Autodesk Inventor part; units mm, degrees
ref_plane "bracket_to_bolt_XY" through (1, 10, 0) normal (0, 0, 1) x (1, 0, 0)
ref_plane "bracket_to_bolt_YZ" through (1, 10, 0) normal (1, 0, 0) x (0, 1, 0)
ref_plane "bracket_to_bolt_ZX" through (1, 10, 0) normal (0, 1, 0) x (0, 0, 1)
sketch "Sketch_15" plane through (0, 0, 0) normal (1, 0, 0) x (0, 1, 0)
  line L0 (4.0858, 30) -> (0, 30)
  line L1 (0, 30) -> (0, 0)
  line L2 (0, 0) -> (30, 0)
  line L3 (30, 0) -> (30, 4.0858)
  arc A0 (30, 4.0858) -> (29.7071, 4.7929) centre (29, 4.0858) ccw
  line L4 (29.7071, 4.7929) -> (4.7929, 29.7071)
  arc A1 (4.7929, 29.7071) -> (4.0858, 30) centre (4.0858, 29) ccw
extrude "Extrusion1" add sketch "Sketch_15" along normal mid plane 20
sketch "Sketch_16" plane through (0, 0, 0) normal (1, 0, 0) x (0, 1, 0)
  line L0 (34.5, 34.5) -> (2.9278, 34.5)
  line L1 (2.9278, 34.5) -> (4.5, 4.5)
  line L2 (4.5, 4.5) -> (34.5, 4.5)
  line L3 (34.5, 4.5) -> (34.5, 34.5)
extrude "Extrusion2" cut sketch "Sketch_16" along normal mid plane 15
sketch "Sketch_17" plane through (0, 4.5, 0) normal (0, 1, 0) x (1, 0, 0)
  line L0 (-5.4209, -10.5) -> (-4.4687, -18.5299)
  arc A0 (-4.4687, -18.5299) -> (4.4687, -18.5299) centre (0, -18) ccw
  line L1 (4.4687, -18.5299) -> (5.4209, -10.5)
  line L2 (5.4209, -10.5) -> (-5.4209, -10.5)
extrude "Extrusion3" add sketch "Sketch_17" against normal blind 2.25
sketch "Sketch_18" plane through (0, 12, 0) normal (0, 1, 0) x (1, 0, 0)
  line L0 (7.5, -12) -> (10, -12)
  line L1 (10, -12) -> (10, -14.5)
  line L2 (10, -14.5) -> (9.567, -14.067)
  line L3 (9.567, -14.067) -> (7.933, -14.067)
  line L4 (7.933, -14.067) -> (7.5, -14.5)
  line L5 (7.5, -14.5) -> (7.5, -12)
  line L6 (7.5, -12) -> (10, -12)
revolve "Revolution1" cut sketch "Sketch_18" angle 360 about axis through (7.5, 12, 12) along (-1, 0, 0)
thread "Thread1"
sketch "Sketch_19" plane through (0, 12, 0) normal (0, 1, 0) x (1, 0, 0)
  line L0 (-10, -12) -> (-7.5, -12)
  line L1 (-7.5, -12) -> (-7.5, -14.5)
  line L2 (-7.5, -14.5) -> (-7.933, -14.067)
  line L3 (-7.933, -14.067) -> (-9.567, -14.067)
  line L4 (-9.567, -14.067) -> (-10, -14.5)
  line L5 (-10, -14.5) -> (-10, -12)
  line L6 (-10, -12) -> (-7.5, -12)
revolve "Revolution2" cut sketch "Sketch_19" angle 360 about axis through (-10, 12, 12) along (-1, 0, 0)
thread "Thread2"
sketch "Sketch6" plane through (10, 30, 0) normal (0, 0, -1) x (-1, 0, 0)
  point P0 (10, -12)
hole "Hole1" at (0, 18, 0) direction (0, 0, 1) diameter 5.2 depth 4.5
sketch "Sketch7" plane through (10, 30, 0) normal (0, 0, -1) x (-1, 0, 0)
  point P0 (10, -20)
hole "Hole2" at (0, 10, 0) direction (0, 0, 1) diameter 5.2 depth 4.5
sketch "Sketch8" plane through (-10, 0, 0) normal (0, -1, 0) x (1, 0, 0)
  point P0 (10, 18)
hole "Hole3" at (0, 0, 18) direction (0, 1, 0) diameter 5.2 depth 4.5
sketch "Sketch_1" plane through (0, 0, 0) normal (0, 1, 0) x (-1, 0, 0)
  line L0 (10, 30) -> (-10, 30)
  line L1 (-10, 30) -> (-10, 0)
  line L2 (-10, 0) -> (10, 0)
  line L3 (10, 0) -> (10, 30)
extrude "Extrusion4" add sketch "Sketch_1" against normal blind 1
sketch "Sketch_4" plane through (0, 0, 0) normal (0, 1, 0) x (-1, 0, 0)
  line L0 (10, 30) -> (-10, 30)
  line L1 (-10, 30) -> (-10, 0)
  line L2 (-10, 0) -> (10, 0)
  line L3 (10, 0) -> (10, 30)
  line L4 (3, 24.3) -> (3, 26.7)
  arc A0 (3, 26.7) -> (2.7, 27) centre (2.7, 26.7) ccw
  line L5 (2.7, 27) -> (-2.7, 27)
  arc A1 (-2.7, 27) -> (-3, 26.7) centre (-2.7, 26.7) ccw
  line L6 (-3, 26.7) -> (-3, 24.3)
  arc A2 (-3, 24.3) -> (-2.7, 24) centre (-2.7, 24.3) ccw
  line L7 (-2.7, 24) -> (2.7, 24)
  arc A3 (2.7, 24) -> (3, 24.3) centre (2.7, 24.3) ccw
  line L8 (3, 5.3) -> (3, 10.7)
  arc A4 (3, 10.7) -> (2.7, 11) centre (2.7, 10.7) ccw
  line L9 (2.7, 11) -> (-2.7, 11)
  arc A5 (-2.7, 11) -> (-3, 10.7) centre (-2.7, 10.7) ccw
  line L10 (-3, 10.7) -> (-3, 5.3)
  arc A6 (-3, 5.3) -> (-2.7, 5) centre (-2.7, 5.3) ccw
  line L11 (-2.7, 5) -> (2.7, 5)
  arc A7 (2.7, 5) -> (3, 5.3) centre (2.7, 5.3) ccw
extrude "Extrusion5" cut sketch "Sketch_4" against normal blind 1
ref_plane "bracket_to_bolt_XY" through (1, 10, 0) normal (0, 0, 1) x (1, 0, 0)
ref_plane "bracket_to_bolt_YZ" through (1, 10, 0) normal (1, 0, 0) x (0, 1, 0)
ref_plane "bracket_to_bolt_ZX" through (1, 10, 0) normal (0, 1, 0) x (0, 0, 1)
ref_plane "bracket_to_dummy_XY" through (0, 0, 0) normal (0, 1, 0) x (1, 0, 0)
ref_plane "bracket_to_dummy_YZ" through (0, 0, 0) normal (1, 0, 0) x (0, 0, -1)
ref_plane "bracket_to_dummy_ZX" through (0, 0, 0) normal (0, 0, -1) x (0, 1, 0)
ref_plane "to_bolt_4_7_base_XY" through (0, 4.5, 18) normal (0, 1, 0) x (1, 0, 0)
ref_plane "to_bolt_4_7_base_YZ" through (0, 4.5, 18) normal (1, 0, 0) x (0, 0, -1)
ref_plane "to_bolt_4_7_base_ZX" through (0, 4.5, 18) normal (0, 0, -1) x (0, 1, 0)
ref_plane "to_bolt_row_4_to_7_XY" through (0, 18, 4.5) normal (0, 0, 1) x (1, 0, 0)
ref_plane "to_bolt_row_4_to_7_YZ" through (0, 18, 4.5) normal (1, 0, 0) x (0, 1, 0)
ref_plane "to_bolt_row_4_to_7_ZX" through (0, 18, 4.5) normal (0, 1, 0) x (0, 0, 1)
ref_plane "to_nut_base_4_7_XY" through (0, -2, 18) normal (0, 1, 0) x (1, 0, 0)
ref_plane "to_nut_base_4_7_YZ" through (0, -2, 18) normal (1, 0, 0) x (0, 0, -1)
ref_plane "to_nut_base_4_7_ZX" through (0, -2, 18) normal (0, 0, -1) x (0, 1, 0)
ref_plane "to_nut_row_4_to_7_XY" through (0, 18, -2) normal (0, 0, 1) x (1, 0, 0)
ref_plane "to_nut_row_4_to_7_YZ" through (0, 18, -2) normal (1, 0, 0) x (0, 1, 0)
ref_plane "to_nut_row_4_to_7_ZX" through (0, 18, -2) normal (0, 1, 0) x (0, 0, 1)
properties part number "HBLFSNK5-C-SEPh5"
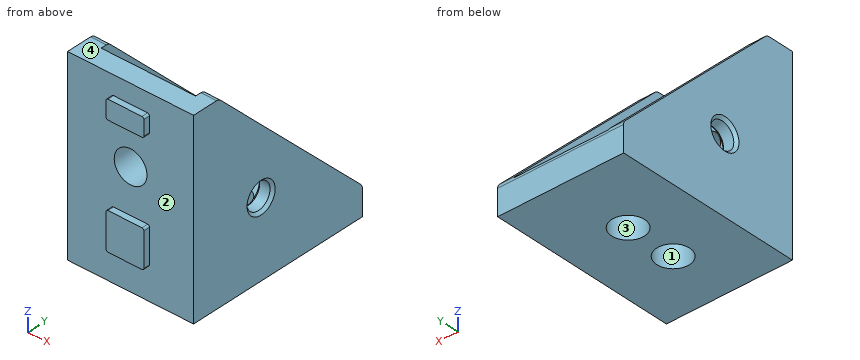
For this review, take the finished solid that the model builds, in its own axes (mm). Face numbers are marked on the shaded views. Round coordinates to 2 decimals unless told otherwise and drop trailing zeros. Write each loop counter-clockwise with the first axis right and the second up, starting at its lowest first coordinate (ties: lowest second). Pieces come first, ordered by that corner, then holes. Notation, with made-up numbers: (58.25, 28) - (111.25, 28) arc R6 ccw to (111.25, 34) - close; hole circle Ø6 at (49, -15.5). An arc over 180 degrees is marked (long way). Write each question's results on one line, items separated by ' | '.
Item 1: Take a section at D-D on y = 2.5. State the section outline as (x, z) points, then the cut area to 3 significant figures.
Calculated:
outline: (-10, 0) - (10, 0) - (10, 30) - (-10, 30) - close; hole circle Ø5.2 at (0, 18) | area: 579 mm^2
Item 2: Take a section at C-C on z = 19.25. State the section outline as (x, y) points, then the cut area to 3 significant figures.
Calculated:
outline: (-10, 0) - (-2.28, 0) - (-2.28, 4.5) - (-4.32, 4.5) - (-4.32, 3.73) - (-7.5, 3.73) - (-7.5, 15.25) - (-10, 15.25) - close; (2.28, 0) - (10, 0) - (10, 15.25) - (7.5, 15.25) - (7.5, 3.73) - (4.32, 3.73) - (4.32, 4.5) - (2.28, 4.5) - close | area: 118 mm^2
Item 3: Take a section at A-A on x = 0. Count the separate pieces of the cut face and the enclosed holes in it, then the cut area to 3 significant figures.
Calculated:
separate pieces: 4 | enclosed holes: 0 | area: 179 mm^2
Item 4: Draft analysis for pull direction Y (two halves, no side actions). For the marked faces 1, 2, 3 and 4, state which applies: pulls with the +Y half, pulls with the -Y half, needs draft (parallel to the pull), parting line crosses it, or undercut.
Calculated:
face 1: undercut | face 2: pulls with the -Y half | face 3: undercut | face 4: needs draft
Item 5: Take a section at B-B on y = 18. State the section outline as (x, z) points.
Calculated:
outline: (-10, 0) - (-2.6, 0) - (-2.6, 4.5) - (-7.5, 4.5) - (-7.5, 16.5) - (-10, 16.5) - close; (2.6, 0) - (10, 0) - (10, 16.5) - (7.5, 16.5) - (7.5, 4.5) - (2.6, 4.5) - close
Item 6: For pin 1 (5 mm diameter, centred on x = 7, y = 12, fed in from -Z); pin 2 (0.5 mm diameter, centred on x = -1, y = -0.5, fed in from +Z); pin 3 (0.8 mm diameter, centred on y = -0.5, z = 8, fed in from +X); pin 4 (6 mm diameter, centred on x = 0, z = 18, fed in from +Y), all flat-tipped, find the tip position at first contact; note any pin that passes through.
Calculated:
pin 1: stops at z = 0 | pin 2: stops at z = 27 | pin 3: stops at x = 3 | pin 4: stops at y = 4.5
Item 7: To check wall thickness, follow line 1 along Y through (x, z) = (0, 1.9); line 2 along X through (y, z) = (2.6, 18); line 3 along Y through (x, z) = (8.8, 12). State the ranges of each line that lie inside material, in increasing order. Write a range as from..to.
Calculated:
line 1: y = 0..7.4, 12.6..15.4, 20.6..30 | line 2: x = -10..-2.6, 2.6..10 | line 3: y = 0..9.93, 14.07..22.5
